Check sheet for the modelled part. Datum: model origin and axes. Units: mm. A direction names the side the tool comes from. Coordinates: 2 decimals unless noted, no trailing zeros. Order: outer loops, then holes, each group sorted by start corner. A loop starts at its lowest first (then second) coordinate and runs counter-clockwise, first axis right, second up.
1. Thickness scan on line 1 (Z direction, x = 21, y = 1.15); line 2 (Z direction, x = 5, y = 2.3); line 3 (X direction, y = 0.7, z = 16). Record the ranges inside material, lowest first.
2. Draft check along X on faces 4 (the flat face through (23, 1, 32.5)), 5 (the flat face through (27.5, 1, 0)), 6 (the cylindrical face through (-13, 1, -16)). Enter one of: released by +X, released by -X, zero draft, split by the parting line, or undercut.
3. Gauge pin test, flat ends, axial feed: pin 1 Ø1.5 at (x, y) = (-8.5, 2) entering from -Z; pin 2 Ø1.5 at (y, z) = (1.5, 12) entering from -X; pin 3 Ø1.5 at (x, y) = (7, 2) entering from +Z; pin 4 Ø25 at (x, z) = (5, 0) entering from -Y. Record the tip position at first contact, or that the pin passes through.
4. Cross-section at B-B (z = 0). Enter the section's corners in (x, y), then the cut area to 3 significant figures.
5. Cross-section at D-D (x = 15). Enter the section's corners in (y, z), then the cut area to 3 significant figures.
6. Cross-section at A-A (y = 2.1). Enter the section's corners in (x, z), then the cut area to 3 significant figures.
7. Set-up check for faces 1 (the flat face through (4, 2, 23.508)), 2 (the flat face through (0, 1, -29.5)), 3 (the flat face through (0, 1, 29.5)): record each of +Z, -Z, +X, -X, +Y, -Y from which the full face is reachable in a straight line by a thin tool's end or side.
8. Cross-section at C-C (x = 5). Enter the section's corners in (y, z).
Autodesk Inventor part; units mm, degrees
ref_plane "YZ Plane" through (0, 0, 0) normal (1, 0, 0) x (0, 1, 0)
ref_plane "XZ Plane" through (0, 0, 0) normal (0, 1, 0) x (-1, 0, 0)
ref_plane "XY Plane" through (0, 0, 0) normal (0, 0, 1) x (1, 0, 0)
sketch "Sketch1" plane through (0, 0, 0) normal (0, 1, 0) x (-1, 0, 0)
  line L0 (17.5, -29.5) -> (-17.5, -29.5)
  line L1 (-17.5, -29.5) -> (-17.5, -32.5)
  line L2 (-17.5, -32.5) -> (-27.5, -32.5)
  line L3 (-27.5, -32.5) -> (-27.5, 32.5)
  line L4 (-27.5, 32.5) -> (-17.5, 32.5)
  line L5 (-17.5, 32.5) -> (-17.5, 29.5)
  line L6 (-17.5, 29.5) -> (17.5, 29.5)
  line L7 (17.5, -10) -> (19.5, -10)
  line L8 (20.5, -9) -> (20.5, 9)
  line L9 (19.5, 10) -> (17.5, 10)
  line L10 (17.5, 29.5) -> (17.5, 10)
  line L11 (17.5, -10) -> (17.5, -29.5)
  arc A0 (20.5, 9) -> (19.5, 10) centre (19.5, 9) ccw
  arc A1 (19.5, -10) -> (20.5, -9) centre (19.5, -9) ccw
  point P0 (0, 0)
  point P1 (-27.5, 0)
  point P2 (0, -29.5)
  point P3 (20.5, 0)
  dimension "d19" = 59
  dimension "d20" = 45
  dimension "d21" = 10
  dimension "d22" = 3
  dimension "d23" = 20
  dimension "d26" = 2
  dimension "d27" = 3
extrude "Extrusion1" add sketch "Sketch1" along normal blind 3
sketch "Sketch2" plane through (0, 3, 0) normal (0, 1, 0) x (1, 0, 0)
  line L0 (-11, 16) -> (21, 16) construction
  line L1 (-17.5, 29.5) -> (-17.5, 10)
  line L2 (27.5, -32.5) -> (27.5, 32.5)
  line L3 (-17.5, 25.7242) -> (27.5, 25.7242) construction
  point P0 (0, 0)
  point P1 (-11, -16)
  point P2 (21, -16)
  point P3 (5, 25.7242)
  point P4 (5, 16)
  dimension "d7" = 32
  dimension "d8" = 32
  dimension "d10" = 16
hole "Hole1" at (-11, 3, 16) at (-11, 3, -16) at (21, 3, 16) at (21, 3, -16) direction (0, -1, 0) diameter 4 end through all
sketch "Sketch3" plane through (0, 3, 0) normal (0, 1, 0) x (1, 0, 0)
  circle A0 centre (21, -16) radius 2
  circle A1 centre (-11, -16) radius 2
  circle A2 centre (-11, 16) radius 2
  circle A3 centre (21, 16) radius 2
  line L0 (17.5, 29.5) -> (-17.5, 29.5)
  line L1 (-17.5, 29.5) -> (-17.5, 10)
  line L2 (-17.5, 10) -> (-19.5, 10)
  line L3 (-20.5, 9) -> (-20.5, -9)
  line L4 (-19.5, -10) -> (-17.5, -10)
  line L5 (-17.5, -10) -> (-17.5, -29.5)
  line L6 (-17.5, -29.5) -> (17.5, -29.5)
  line L7 (17.5, -29.5) -> (17.5, -32.5)
  line L8 (17.5, -32.5) -> (27.5, -32.5)
  line L9 (27.5, -32.5) -> (27.5, 32.5)
  line L10 (27.5, 32.5) -> (17.5, 32.5)
  line L11 (17.5, 32.5) -> (17.5, 29.5)
  line L12 (-11, 16) -> (21, -16) construction
  line L13 (-11, -16) -> (21, 16) construction
  circle A4 centre (5, 0) radius 15.5278
  arc A5 (-19.5, 10) -> (-20.5, 9) centre (-19.5, 9) ccw
  arc A6 (-20.5, -9) -> (-19.5, -10) centre (-19.5, -9) ccw
  line L14 (-2.9348, -23.5081) -> (10.6481, -23.5081)
  line L15 (10.6481, -20.5081) -> (-2.9348, -20.5081)
  arc A7 (-2.9348, -20.5081) -> (-2.9348, -23.5081) centre (-2.9348, -22.0081) ccw
  arc A8 (10.6481, -23.5081) -> (10.6481, -20.5081) centre (10.6481, -22.0081) ccw
  point P0 (0, 0)
  dimension "d28" = 3
extrude "Extrusion2" cut sketch "Sketch3" against normal up to next contours A4 | A7 L15 A8 L14
equation "\"d27\" = d22"
equation "\"d9\" = 0.5 * d7"
properties part number "Fan_plate" material "Polycarbonate, Smoke"
Data:
1. line 1: z = -32.5 to -18, -14 to 14, 18 to 32.5
1. line 2: z = -29.5 to -15.53, 15.53 to 20.51, 23.51 to 29.5
1. line 3: x = -17.5 to -13, -9 to 19, 23 to 27.5
2. face 4: zero draft
2. face 5: released by +X
2. face 6: undercut
3. pin 1: stops at z = -29.5
3. pin 2: stops at x = -17.5
3. pin 3: stops at z = 29.5
3. pin 4: passes through
4. outline: (-20.5, 0) - (-10.53, 0) - (-10.53, 3) - (-20.5, 3) - close; (20.53, 0) - (27.5, 0) - (27.5, 3) - (20.53, 3) - close
4. area: 50.8 mm2
5. outline: (0, -29.5) - (3, -29.5) - (3, -11.88) - (0, -11.88) - close; (0, 11.88) - (3, 11.88) - (3, 29.5) - (0, 29.5) - close
5. area: 106 mm2
6. outline: (-20.5, -9) arc R1 ccw to (-19.5, -10) - (-17.5, -10) - (-17.5, -29.5) - (17.5, -29.5) - (17.5, -32.5) - (27.5, -32.5) - (27.5, 32.5) - (17.5, 32.5) - (17.5, 29.5) - (-17.5, 29.5) - (-17.5, 10) - (-19.5, 10) arc R1 ccw to (-20.5, 9) - close; hole circle Ø4 at (-11, -16); hole circle Ø4 at (-11, 16); hole circle Ø31.06 at (5, 0); hole (-2.93, 20.51) - (10.65, 20.51) arc R1.5 ccw to (10.65, 23.51) - (-2.93, 23.51) arc R1.5 ccw to start; hole circle Ø4 at (21, -16); hole circle Ø4 at (21, 16)
6. area: 1,920 mm2
7. face 1: +Y, -Y
7. face 2: -Z, -X, +Y, -Y
7. face 3: +Z, -X, +Y, -Y
8. outline: (0, -29.5) - (3, -29.5) - (3, -15.53) - (0, -15.53) - close; (0, 15.53) - (3, 15.53) - (3, 20.51) - (0, 20.51) - close; (0, 23.51) - (3, 23.51) - (3, 29.5) - (0, 29.5) - close
